Autodesk Fusion 360 part; units mm, degrees
sketch "Esquisse1" plane through (0, 0, 0) normal (0, 0, 1) x (1, 0, 0)
  circle A0 centre (0, 0) radius 1
  dimension "d1" = 2
extrude "Extrusion1" add sketch "Esquisse1" along normal blind 4.3
sketch "Esquisse2" plane through (0, 0, 4.3) normal (0, 0, 1) x (1, 0, 0)
  circle A0 centre (0, 0) radius 1
  circle A1 centre (0, 0) radius 2.25
  dimension "d4" = 4.5
extrude "Extrusion2" add sketch "Esquisse2" along normal blind 1.2 contours A0 | A1
sketch "Esquisse3" plane through (0, 0, 5.5) normal (0, 0, 1) x (1, 0, 0)
  circle A0 centre (0, 0) radius 2.25
  circle A1 centre (0, 0) radius 1.55
  dimension "d7" = 3.1
extrude "Extrusion3" add sketch "Esquisse3" along normal blind 8.7 contours A1
extrude "Extrusion4" cut 1 faces at (-0.3296, 0.5031, 0) along direction (0, 0, 1) blind 4.3
extrude "Extrude5" cut 1 faces at (0.8338, -0.7144, 14.2) along direction (0, 0, -1) blind 0.5
fillet "Fillet2" radius 1.55 1 edges at (-1.4451, 0.5605, 13.7)
Geometry: final body of the model. Coordinates: model frame, mm. A direction names the side the tool comes from. Give positions to 0.01 mm unless a question says otherwise; leave off trailing zeros. Loops run counter-clockwise (first coordinate to the right, second up) from the corner with the lowest first, then second, coordinate; pieces in that order, holes last. Notation, with made-up numbers: M 56,87 L 106,87 A30 cw 106,115 Z; hole C -4,-36.75 d6. An arc over 180 degrees is marked long. Put each result on its own line as item: value.
1) Cut plane C-C, the plane z = 10.25. Return the cut outline in (x, y), plus the area to 3 significant figures.
Computed values:
outline: C 0,0 d3.1
area: 7.55 mm^2
2) Reachability of faces 1 (the flat face through (-2, 0, 5.5)), 2 (the cylindrical face through (-0.29, -2.23, 4.89)) from +Z, -Z, +X, -X, +Y, -Y: full face, straight path, thin tool, end or side. Return the list, or none.
Computed values:
face 1: +Z
face 2: +Z, -Z
3) Cut plane A-A, the plane y = 0. Return the cut outline in (x, z).
Computed values:
outline: M -2.25,4.3 L 2.25,4.3 L 2.25,5.5 L 1.55,5.5 L 1.55,12.15 A1.55 ccw -1.55,12.15 L -1.55,5.5 L -2.25,5.5 Z
4) Cut plane D-D, the plane z = 12.25. Return the cut outline in (x, y).
Computed values:
outline: C 0,0 d3.09
5) First-contact query: P1, Ø2, axis at x = 1, z = 10.5, coming from the +Y side; P2, Ø2, axis at x = -0.5, y = 1.5, coming from the +Z side. Flat tips, straight axial feed; report the tip coordinate or a pass-through.
Computed values:
P1: stops at y = 1.55
P2: stops at z = 13.59
6) Material intervals for L1, parallel to Z at x = 0.85, y = -1.75; L2, parallel to Y at x = 0.9, z = 7.5; L3, parallel to X at y = -1.3, z = 11, sorted ascending. Write a range as from..to.
Computed values:
L1: z = 4.3..5.5
L2: y = -1.26..1.26
L3: x = -0.84..0.84
